```python
from build123d import *

# Parameters (mm, degrees)
SURFACE_EXTRUDE1_1_DEPTH = 2.5
THICKEN1_T1              = 0.4
SKETCH2_W                = 0.4
SKETCH2_H                = 3.67
BOSS_EXTRUDE1_DEPTH      = 4.5
CUT_EXTRUDE1_REACH       = 13.776
SKETCH3_W                = 3.4
SKETCH3_H                = 1
FILLET2_RADIUS           = 1.335
FILLET2_LENGTH           = 0.4


with BuildPart() as body_1:
    # Surface-Extrude1: a surface, the sketch's curves swept straight by 2.5 mm
    with BuildLine(Plane.XY, mode=Mode.PRIVATE) as surface_extrude1_1_path:
        Line((-7.064526383, 1.105941224), (-2.1639905, -1.391006524))
        ThreePointArc((-2.1639905, -1.391006524), (-1.187501435, -1.352640164), (-0.71, -0.5))
        Line((-0.71, -0.5), (-0.71, 0))
        Line((-0.71, 0), (-0.71, 3.67))
        ThreePointArc((-0.71, 3.67), (0, 4.38), (0.71, 3.67))
        Line((0.71, 3.67), (0.71, 0))
    surface_extrude1_1 = Shell.extrude(surface_extrude1_1_path.wire(), (0 * SURFACE_EXTRUDE1_1_DEPTH, 0 * SURFACE_EXTRUDE1_1_DEPTH, 1 * SURFACE_EXTRUDE1_1_DEPTH))
    add(Solid.thicken(surface_extrude1_1, THICKEN1_T1))

    # Sketch2 → Boss-Extrude1 (add)
    with BuildSketch(Plane.XY.offset(2.5)):
        with Locations((0.91, 1.835)):
            Rectangle(SKETCH2_W, SKETCH2_H)
    extrude(amount=BOSS_EXTRUDE1_DEPTH)

    # Sketch3 → Cut-Extrude1 (cut, up to next)
    with BuildSketch(Plane(origin=(1.11, 0, 0), x_dir=(0, 0, -1), z_dir=(1, 0, 0)), mode=Mode.PRIVATE) as cut_extrude1_sk1:
        with Locations((-5.3, 0.5)):
            Rectangle(SKETCH3_W, SKETCH3_H)
    cut_extrude1_tool1 = extrude(cut_extrude1_sk1.sketch, amount=-CUT_EXTRUDE1_REACH, mode=Mode.PRIVATE) & body_1.part
    add(cut_extrude1_tool1.solids().sort_by_distance((1.11, 0.5, 5.3))[0], mode=Mode.SUBTRACT)

    # Fillet2: full round fillet: the end face becomes a half cylinder, R = half its width
    fillet2_face = Plane((0.91, 2.335, 7), x_dir=(-1, 0, 0), z_dir=(0, 0, 1))  # on the end face: x along it, z out of the body
    fillet2_slab = fillet2_face.offset(-FILLET2_RADIUS / 2) * Box(FILLET2_LENGTH, 2 * FILLET2_RADIUS, FILLET2_RADIUS, mode=Mode.PRIVATE)  # the body's end, R deep
    fillet2_round = Plane((0.91, 2.335, 5.665), x_dir=(0, 0, 1), z_dir=(-1, 0, 0)) * Cylinder(FILLET2_RADIUS, FILLET2_LENGTH, mode=Mode.PRIVATE)  # its axis R under the face
    add(fillet2_slab - fillet2_round, mode=Mode.SUBTRACT)


solid = body_1.part
```
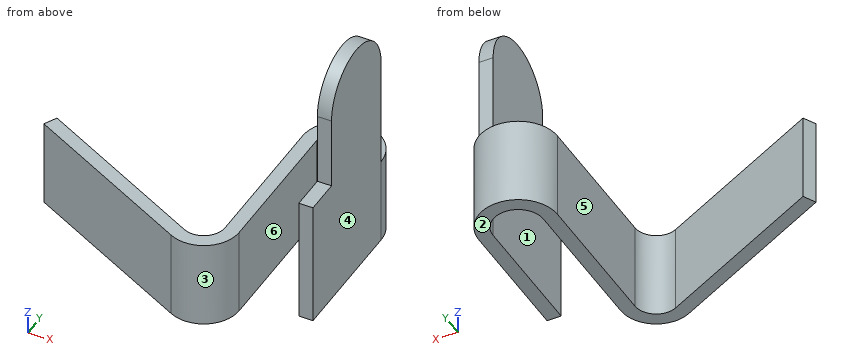
Verification items for the finished model (mm, model axes). Face numbers are marked on the shaded views. A direction names the side the tool comes from. Round coordinates to 2 decimals unless told otherwise and drop trailing zeros. Write each loop counter-clockwise with the first axis right and the second up, starting at its lowest first coordinate (ties: lowest second). Pieces come first, ordered by that corner, then holes. Notation, with made-up numbers: (-24, 72) -> (26, 72) arc R26 cw to (26, 94) -> close; hole circle Ø6 at (6.25, 74). An arc over 180 degrees is marked (long way). Write each question's results on one line, items separated by ' | '. Start each with the question number.
1. Material ranges on probe 1 along X at (y, z) = (2.75, 0.5); probe 2 along Z at (x, y) = (-6.5, 1); probe 3 along X at (y, z) = (3, 2.75), recorded low to high. Write a range as from..to.
2. Draft check along X on the marked faces 1, 2 and 3. Enter one of: +X half, -X half, draft (parallel to the pull), parting line (faces both ways), or undercut.
3. Cross-section at C-C (x = 0). Enter the section's corners in (y, z).
4. Cross-section at A-A (z = 0.75). Enter the section's corners in (x, y), then the cut area to 3 significant figures.
5. Depth check by flat-ended pin: P1, Ø1.5, axis at x = -1.5, y = 4, coming from the +Z side; P2, Ø3, axis at x = -1, z = 5.5, coming from the +Y side; P3, Ø3, axis at y = 2.5, z = 1.5, coming from the -X side. Enter the tip coordinate at first touch or a pass-through.
6. Set-up check for the marked faces 4, 5 and 6: record each of +Z, -Z, +X, -X, +Y, -Y from which the full face is reachable in a straight line by a thin tool's end or side.
7. Cross-section at D-D (z = 3.25). Enter the section's corners in (x, y), then the cut area to 3 significant figures.
8. Cross-section at B-B (y = 4). Enter the section's corners in (x, z).
Solutions:
1) probe 1: x = -1.11..-0.71, 0.71..1.11 | probe 2: z = 0..2.5 | probe 3: x = 0.71..1.11
2) face 1: undercut | face 2: draft | face 3: parting line
3) outline: (4.38, 0) -> (4.78, 0) -> (4.78, 2.5) -> (4.38, 2.5) -> close
4) outline: (-7.06, 1.11) -> (-2.16, -1.39) arc R1 ccw to (-0.71, -0.5) -> (-0.71, 3.67) arc R0.71 cw to (0.71, 3.67) -> (0.71, 0) -> (1.11, 0) -> (1.11, 3.67) arc R1.11 ccw to (-1.11, 3.67) -> (-1.11, -0.5) arc R0.6 cw to (-1.98, -1.03) -> (-6.88, 1.46) -> close | area: 7.13 mm2
5) P1: stops at z = 2.5 | P2: passes through | P3: stops at x = -7.06
6) face 4: +Z, -Z, +X, +Y, -Y | face 5: +Z, -Z, +Y | face 6: +Z, -Z, -Y
7) outline: (0.71, 0) -> (1.11, 0) -> (1.11, 3.67) -> (0.71, 3.67) -> close | area: 1.47 mm2
8) outline: (-1.06, 0) -> (-0.63, 0) -> (-0.63, 2.5) -> (-1.06, 2.5) -> close; (0.63, 0) -> (1.06, 0) -> (1.06, 2.5) -> (0.63, 2.5) -> close
